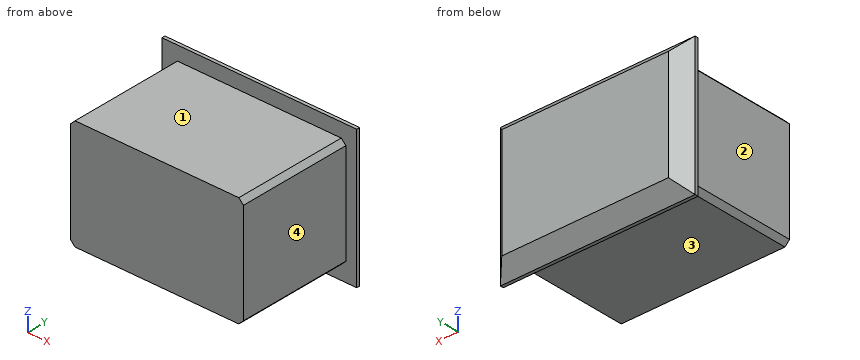
from build123d import *

# Parameters (mm, degrees)
SKETCH1_W           = 18.45
SKETCH1_H           = 11.75
BOSS_EXTRUDE1_DEPTH = 14
SKETCH2_W           = 20.75
SKETCH2_H           = 14.75
BOSS_EXTRUDE2_DEPTH = 1.85
CHAMFER1_SIZE       = 1.5
CHAMFER2_SIZE       = 0.5


with BuildPart() as part:
    # Sketch1 → Boss-Extrude1 (new body)
    with BuildSketch(Plane(origin=(0, 0, 0), x_dir=(1, 0, 0), z_dir=(0, 1, 0))):
        Rectangle(SKETCH1_W, SKETCH1_H)
    extrude(amount=BOSS_EXTRUDE1_DEPTH)

    # Sketch2 → Boss-Extrude2 (add)
    with BuildSketch(Plane(origin=(0, 14, 0), x_dir=(1, 0, 0), z_dir=(0, 1, 0))):
        Rectangle(SKETCH2_W, SKETCH2_H)
    extrude(amount=-BOSS_EXTRUDE2_DEPTH)

    # Chamfer1
    chamfer1_edges = [part.edges().sort_by_distance(p)[0] for p in [
        (-10.375, 14, 0),
        (0, 14, 7.375),
        (10.375, 14, 0),
        (0, 14, -7.375),
    ]]
    chamfer(chamfer1_edges, length=CHAMFER1_SIZE)

    # Chamfer2
    chamfer2_edges = [part.edges().sort_by_distance(p)[0] for p in [
        (-9.225, 6.075, -5.875),
        (9.225, 6.075, -5.875),
        (9.225, 6.075, 5.875),
        (-9.225, 6.075, 5.875),
    ]]
    chamfer(chamfer2_edges, length=CHAMFER2_SIZE)


solid = part.part
Part model, mm, in its own coordinate system. Face numbers are marked on the shaded views. A direction names the side the tool comes from. Coordinates: 2 decimals unless noted, no trailing zeros. Order: outer loops, then holes, each group sorted by start corner. A loop starts at its lowest first (then second) coordinate and runs counter-clockwise, first axis right, second up.
(1) Slice it at B-B, the plane z = -1.5. Write the cut outline in (x, y) (3 decimals), and give its area (3 significant figures).
Check sheet entries:
outline: (-10.375, 12.15) - (-9.225, 12.15) - (-9.225, 0) - (9.225, 0) - (9.225, 12.15) - (10.375, 12.15) - (10.375, 12.5) - (8.875, 14) - (-8.875, 14) - (-10.375, 12.5) - close
area: 260 mm2
(2) Slice it at A-A, the plane y = 4.75. Write the cut outline in (x, z) (3 decimals).
Check sheet entries:
outline: (-9.225, -5.375) - (-8.725, -5.875) - (8.725, -5.875) - (9.225, -5.375) - (9.225, 5.375) - (8.725, 5.875) - (-8.725, 5.875) - (-9.225, 5.375) - close
(3) Probe L1, parallel to X at y = 4.5, z = 4 (3 decimals); L2, parallel to Z at x = -5.5, y = 6.5 (3 decimals); L3, parallel to Y at x = 6.5, z = -6 (3 decimals). List the from-to ranges inside material, lowest first.
Check sheet entries:
L1: x = -9.225 to 9.225
L2: z = -5.875 to 5.875
L3: y = 12.15 to 13.875
(4) Tool access for the marked faces 1, 2, 3 and 4: list every direction of +Z, -Z, +X, -X, +Y, -Y with a clear straight run to the whole face (end or side of a thin tool).
Check sheet entries:
face 1: +Z, +X, -X, -Y
face 2: +Z, -Z, -X, -Y
face 3: -Z, +X, -X, -Y
face 4: +Z, -Z, +X, -Y
(5) Slice it at C-C, the plane x = -4.25. Write the cut outline in (y, z) (3 decimals).
Check sheet entries:
outline: (0, -5.875) - (12.15, -5.875) - (12.15, -7.375) - (12.5, -7.375) - (14, -5.875) - (14, 5.875) - (12.5, 7.375) - (12.15, 7.375) - (12.15, 5.875) - (0, 5.875) - close
(6) Pin check, flat tips, straight feed: pin 1 Ø4 at (y, z) = (8.5, -2) entering from -X (3 decimals); pin 2 Ø2 at (x, y) = (0, 5.5) entering from -Z (3 decimals); pin 3 Ø8 at (y, z) = (6, -1) entering from +X (3 decimals). Stop position of each tip, or through.
Check sheet entries:
pin 1: stops at x = -9.225
pin 2: stops at z = -5.875
pin 3: stops at x = 9.225
